from build123d import *

# Parameters (mm, degrees)
SKETCH2_W                  = 25.4
SKETCH2_H                  = 2.41
BOSS_EXTRUDE1_DEPTH        = 8.51
SKETCH5_W                  = 1
SKETCH5_H                  = 1
CUT_EXTRUDE1_DEPTH         = 5
CHAMFER1_SIZE              = 0.5
LPATTERN3_COUNT            = 10
LPATTERN3_PITCH            = 2.54
CHAMFER1_OF_LPATTERN3_SIZE = 0.5
BOSS_EXTRUDE2_DEPTH        = 11
LPATTERN1_COUNT            = 10
LPATTERN1_PITCH            = 2.54


with BuildPart() as part:
    # Sketch2 → Boss-Extrude1 (new body)
    with BuildSketch(Plane(origin=(0, 0, 0), x_dir=(1, 0, 0), z_dir=(0, 1, 0))):
        with Locations((11.43, 0)):
            Rectangle(SKETCH2_W, SKETCH2_H)
    extrude(amount=BOSS_EXTRUDE1_DEPTH)

    # Sketch5 → Cut-Extrude1 (cut)
    with BuildSketch(Plane(origin=(0, 8.51, 0), x_dir=(1, 0, 0), z_dir=(0, 1, 0))):
        Rectangle(SKETCH5_W, SKETCH5_H)
    cut_extrude1 = extrude(amount=-CUT_EXTRUDE1_DEPTH, mode=Mode.SUBTRACT)

    # Chamfer1
    chamfer1_edges = [part.edges().sort_by_distance(p)[0] for p in [
        (0.5, 8.51, 0),
        (0, 8.51, -0.5),
        (-0.5, 8.51, 0),
        (0, 8.51, 0.5),
    ]]
    chamfer(chamfer1_edges, length=CHAMFER1_SIZE)

    # LPattern3: Cut-Extrude1 ×10
    with Locations(*[(i * LPATTERN3_PITCH, 0, 0) for i in range(1, LPATTERN3_COUNT)]):
        add(cut_extrude1, mode=Mode.SUBTRACT)

    # Chamfer1 of LPattern3
    chamfer1_of_lpattern3_edges = [part.edges().sort_by_distance(p)[0] for p in [
        (3.04, 8.51, 0),
        (2.54, 8.51, -0.5),
        (2.04, 8.51, 0),
        (2.54, 8.51, 0.5),
        (5.58, 8.51, 0),
        (5.08, 8.51, -0.5),
        (4.58, 8.51, 0),
        (5.08, 8.51, 0.5),
        (8.12, 8.51, 0),
        (7.62, 8.51, -0.5),
        (7.12, 8.51, 0),
        (7.62, 8.51, 0.5),
        (10.66, 8.51, 0),
        (10.16, 8.51, -0.5),
        (9.66, 8.51, 0),
        (10.16, 8.51, 0.5),
        (13.2, 8.51, 0),
        (12.7, 8.51, -0.5),
        (12.2, 8.51, 0),
        (12.7, 8.51, 0.5),
        (15.74, 8.51, 0),
        (15.24, 8.51, -0.5),
        (14.74, 8.51, 0),
        (15.24, 8.51, 0.5),
        (18.28, 8.51, 0),
        (17.78, 8.51, -0.5),
        (17.28, 8.51, 0),
        (17.78, 8.51, 0.5),
        (20.82, 8.51, 0),
        (20.32, 8.51, -0.5),
        (19.82, 8.51, 0),
        (20.32, 8.51, 0.5),
        (23.36, 8.51, 0),
        (22.86, 8.51, -0.5),
        (22.36, 8.51, 0),
        (22.86, 8.51, 0.5),
    ]]
    chamfer(chamfer1_of_lpattern3_edges, length=CHAMFER1_OF_LPATTERN3_SIZE)

    # Sketch8 → Boss-Extrude2 (add)
    with BuildSketch(Plane(origin=(0, 0, 0), x_dir=(1, 0, 0), z_dir=(0, 1, 0))):
        with BuildLine():
            Line((-0.3, -0.2), (0.3, -0.2))
            ThreePointArc((0.3, -0.2), (0.370710678, -0.170710678), (0.4, -0.1))
            Line((0.4, -0.1), (0.4, 0.1))
            ThreePointArc((0.4, 0.1), (0.370710678, 0.170710678), (0.3, 0.2))
            Line((0.3, 0.2), (-0.3, 0.2))
            ThreePointArc((-0.3, 0.2), (-0.370710678, 0.170710678), (-0.4, 0.1))
            Line((-0.4, 0.1), (-0.4, -0.1))
            ThreePointArc((-0.4, -0.1), (-0.370710678, -0.170710678), (-0.3, -0.2))
        make_face()
    boss_extrude2 = extrude(amount=-BOSS_EXTRUDE2_DEPTH)

    # LPattern1: Boss-Extrude2 ×10
    with Locations(*[(i * LPATTERN1_PITCH, 0, 0) for i in range(1, LPATTERN1_COUNT)]):
        add(boss_extrude2)


solid = part.part
Design review of the part built by this model. Coordinates are the model's own, in mm. Round coordinates to 2 decimals unless told otherwise and drop trailing zeros. Loops run counter-clockwise (first coordinate to the right, second up) from the corner with the lowest first, then second, coordinate; pieces in that order, holes last. Notation, with made-up numbers: (-7.75, 40.5) - (-1.75, 40.5) arc R17 ccw to (-1.75, 71.5) - close; hole circle Ø2 at (82.5, 54.5). An arc over 180 degrees is marked (long way). One line per item, written item: value. Start each with the question number.
1) Consider section B-B on x = 15.25. Give the boundary of the cut face in (y, z) (3 decimals).
2) To check wall thickness, follow L1, parallel to Z at x = 10.25, y = 6.5 (3 decimals); L2, parallel to Z at x = 5.25, y = -9; L3, parallel to Y at x = 9, z = 0.1. State the ranges of each line that lie inside material, in increasing order. Write a range as from..to.
3) Draft analysis for pull direction X (two halves, no side actions). For faces 1 (the flat face through (20.82, 6, 0)), 2 (the flat face through (7.6, 5.8, 0.5)), 3 (the flat face through (24.13, 4, 0)), state which applies: +X half, -X half, draft (parallel to the pull), parting line (faces both ways), or undercut.
4) Consider section A-A on y = -10. Give the number of separate pieces and of enclosed holes in the cut face, then the cut area to 3 significant figures.
5) Insertion check: pin 1 Ø0.7 at (x, y) = (18, -6.5) entering from -Z; pin 2 Ø0.5 at (x, z) = (12.5, 0) entering from +Y. Each pin has a flat end and moves straight along its axis. Give the tip position at first contact, or say it passes through.
Reported:
1. outline: (-11, -0.2) - (0, -0.2) - (0, -1.205) - (8.51, -1.205) - (8.51, -1) - (8.01, -0.5) - (3.51, -0.5) - (3.51, 0.5) - (8.01, 0.5) - (8.51, 1) - (8.51, 1.205) - (0, 1.205) - (0, 0.2) - (-11, 0.2) - close
2. L1: z = -1.205..-0.5, 0.5..1.205
2. L2: z = -0.2..0.2
2. L3: y = 0..8.51
3. face 1: undercut
3. face 2: undercut
3. face 3: +X half
4. separate pieces: 10
4. enclosed holes: 0
4. area: 3.11 mm^2
5. pin 1: stops at z = -0.2
5. pin 2: stops at y = 3.51
